Check sheet for the modelled part. Datum: model origin and axes. Units: mm. Give positions to 0.01 mm unless a question says otherwise; leave off trailing zeros. Write each loop counter-clockwise with the first axis right and the second up, starting at its lowest first coordinate (ties: lowest second). Pieces come first, ordered by that corner, then holes. Notation, with made-up numbers: (18, 84.25) -> (76, 84.25) arc R14 cw to (76, 105.25) -> close; hole circle Ø11 at (-22.75, 47). An arc over 180 degrees is marked (long way). Answer as a JSON object with one key per item and string values.
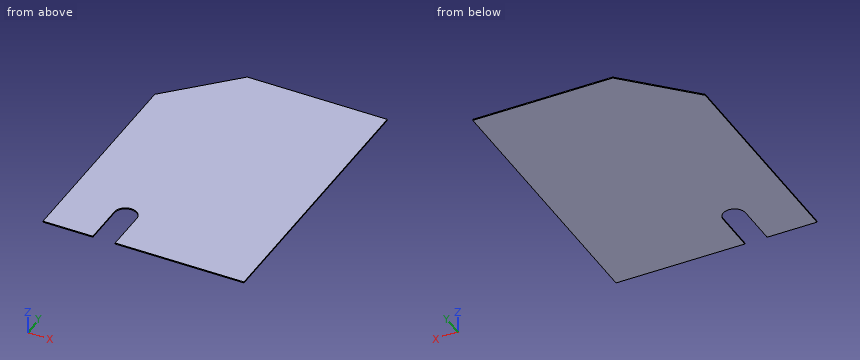
from build123d import *

# Parameters (mm, degrees)
SM_BASE_FLANGE_1_DEPTH = 1.5


# Sheet-metal steps are written as plain solids
with BuildPart() as part:
    # Sketch 1 → Базовая кромка1 (new body)
    with BuildSketch(Plane.XY):
        with BuildLine():
            Line((-270.076706029, 290.501117881), (-270.076706029, 0))
            Line((-270.076706029, 0), (-203.076706029, 0))
            Line((-203.076706029, 0), (-203.076706029, 55.811778053))
            ThreePointArc((-203.076706029, 55.811778053), (-188.076706029, 70.811778053), (-173.076706029, 55.811778053))
            Line((-173.076706029, 55.811778053), (-173.076706029, 0))
            Line((-173.076706029, 0), (0, 0))
            Line((0, 0), (0, 372.061778053))
            ThreePointArc((0, 372.061778053), (-0.219669914, 372.592108139), (-0.75, 372.811778053))
            Line((-0.75, 372.811778053), (-187.766045857, 372.811778053))
            ThreePointArc((-187.766045857, 372.811778053), (-188.053058432, 372.754687702), (-188.296375943, 372.592108139))
            Line((-188.296375943, 372.592108139), (-269.857036115, 291.031447967))
            ThreePointArc((-269.857036115, 291.031447967), (-270.019615678, 290.788130455), (-270.076706029, 290.501117881))
        make_face()
    extrude(amount=-SM_BASE_FLANGE_1_DEPTH)


solid = part.part
1. Sectioned sample at A-A, the plane y = 28.5. Enter the section's corners in (x, z).
Determined:
{"outline": "(-270.08, -1.5) -> (-203.08, -1.5) -> (-203.08, 0) -> (-270.08, 0) -> close; (-173.08, -1.5) -> (0, -1.5) -> (0, 0) -> (-173.08, 0) -> close"}
2. Scan lines: L1, parallel to X at y = 57, z = -0.6; L2, parallel to X at y = 47, z = -0.4; L3, parallel to Y at x = -236.5, z = -0.45. Record each from-to range of solid material in increasing order. Write a range as [from, to].
Determined:
{"L1": "[-270.08, -203.03], [-173.12, 0]", "L2": "[-270.08, -203.08], [-173.08, 0]", "L3": "[0, 324.39]"}
3. Sectioned sample at B-B, the plane z = -1.1. Enter the section's corners in (x, y), plus the area to 3 significant figures.
Determined:
{"outline": "(-270.08, 0) -> (-203.08, 0) -> (-203.08, 55.81) arc R15 cw to (-173.08, 55.81) -> (-173.08, 0) -> (0, 0) -> (0, 372.06) arc R0.75 ccw to (-0.75, 372.81) -> (-187.77, 372.81) arc R0.75 ccw to (-188.3, 372.59) -> (-269.86, 291.03) arc R0.75 ccw to (-270.08, 290.5) -> close", "area": "95,300 mm^2"}
4. Sectioned sample at C-C, the plane x = -226. Enter the section's corners in (y, z), plus the area to 3 significant figures.
Determined:
{"outline": "(0, -1.5) -> (334.89, -1.5) -> (334.89, 0) -> (0, 0) -> close", "area": "502 mm^2"}
